Design review of the part built by this model. Coordinates are the model's own, in mm. A direction names the side the tool comes from. Give positions to 0.01 mm unless a question says otherwise; leave off trailing zeros. Order: outer loops, then holes, each group sorted by start corner. A loop starts at its lowest first (then second) coordinate and runs counter-clockwise, first axis right, second up.
```python
from build123d import *

# Parameters (mm, degrees)
BOSS_EXTRUDE1_DEPTH          = 75
SKETCH2_R                    = 2
CUT_EXTRUDE1_DEPTH           = 15
SKETCH4_R                    = 2
CUT_EXTRUDE2_DEPTH           = 12
SKETCH3_R                    = 2.3876
CUT_EXTRUDE3_DEPTH           = 6.35
CUT_EXTRUDE3_DRAFT           = -8
CUT_EXTRUDE3_PROFILE_2_DEPTH = 6.35
CUT_EXTRUDE3_PROFILE_2_DRAFT = -8
CUT_EXTRUDE4_START           = -3
CUT_EXTRUDE4_DEPTH           = 3
CUT_EXTRUDE5_START           = -3
CUT_EXTRUDE5_DEPTH           = 3
CUT_EXTRUDE6_START           = -3
CUT_EXTRUDE6_DEPTH           = 3
CUT_EXTRUDE7_START           = -3
CUT_EXTRUDE7_DEPTH           = 3
SKETCH9_R                    = 1.4951657
CUT_EXTRUDE8_DEPTH           = 5
MIRROR2_COPY_1_SKETCH_R      = 2.3876
MIRROR2_COPY_1_DEPTH         = 6.35
MIRROR2_COPY_1_DRAFT         = -8
MIRROR2_COPY_2_SKETCH_R      = 2.3876
MIRROR2_COPY_2_DEPTH         = 6.35
MIRROR2_COPY_2_DRAFT         = -8
MIRROR2_COPY_3_SKETCH_R      = 2.3876
MIRROR2_COPY_3_DEPTH         = 6.35
MIRROR2_COPY_3_DRAFT         = -8
FILLET2_START                = 5.175
FILLET2_DEPTH                = 42.1845
FILLET2_START_2              = 10.175
FILLET2_2_DEPTH              = 3.491666667
FILLET2_3_DEPTH              = 37.825
FILLET3_R                    = 2


with BuildPart() as part:
    # Sketch1 → Boss-Extrude1 (new body)
    with BuildSketch(Plane(origin=(0, 0, 0), x_dir=(1, 0, 0), z_dir=(0, 1, 0))):
        with BuildLine():
            Line((-6.825, -6.666666667), (-6.825, -25.333333333))
            Line((-6.825, -25.333333333), (8.175, -25.333333333))
            Line((8.175, -25.333333333), (8.175, -13.175))
            Line((8.175, -13.175), (55, -13.175))
            Line((55, -13.175), (55, -1.175))
            Line((55, -1.175), (25, -1.175))
            Line((25, -1.175), (25, 2))
            ThreePointArc((25, 2), (14.923352523, 3.572976633), (5.805515239, 8.142235123))
            ThreePointArc((5.805515239, 8.142235123), (3.047757271, 9.524241472), (0, 10))
            ThreePointArc((0, 10), (-7.071067812, 7.071067812), (-10, 0))
            Line((-10, 0), (-10, -6.666666667))
            Line((-10, -6.666666667), (-6.825, -6.666666667))
        make_face()
    extrude(amount=BOSS_EXTRUDE1_DEPTH)

    # Sketch2 → Cut-Extrude1 (cut)
    with BuildSketch(Plane.ZY.offset(6.825)):
        with Locations((15.666666667, 65)):
            Circle(SKETCH2_R)
    cut_extrude1 = extrude(amount=-CUT_EXTRUDE1_DEPTH, mode=Mode.SUBTRACT)

    # Sketch4 → Cut-Extrude2 (cut)
    with BuildSketch(Plane(origin=(0, 0, 1.175), x_dir=(-1, 0, 0), z_dir=(0, 0, -1))):
        with Locations((-45, 65)):
            Circle(SKETCH4_R)
    cut_extrude2 = extrude(amount=-CUT_EXTRUDE2_DEPTH, mode=Mode.SUBTRACT)


with BuildPart() as cut_extrude3_tool:
    # Sketch3 → Cut-Extrude3 (with draft: the straight prism first)
    with BuildSketch(Plane(origin=(0, 75, 0), x_dir=(1, 0, 0), z_dir=(0, 1, 0))):
        with Locations((1, -1)):
            Circle(SKETCH3_R)
    extrude(amount=-CUT_EXTRUDE3_DEPTH)
    # Cut-Extrude3: the draft: its side faces are tilted about the plane it starts from
    cut_extrude3_sides = [cut_extrude3_tool.faces().sort_by_distance(p)[0] for p in [
        (-1.3876, 71.825, 1),
    ]]
    draft(cut_extrude3_sides, Plane(origin=(0, 75, 0), x_dir=(1, 0, 0), z_dir=(0, 1, 0)), CUT_EXTRUDE3_DRAFT)


with BuildPart() as part_1:
    add(part.part)

    # Cut-Extrude3: cut by cut_extrude3_tool
    add(cut_extrude3_tool.part, mode=Mode.SUBTRACT)


with BuildPart() as cut_extrude3_profile_2_tool:
    # Sketch3 → Cut-Extrude3 profile 2 (with draft: the straight prism first)
    with BuildSketch(Plane(origin=(0, 75, 0), x_dir=(1, 0, 0), z_dir=(0, 1, 0))):
        with Locations((30, -7.175)):
            Circle(SKETCH3_R)
    extrude(amount=-CUT_EXTRUDE3_PROFILE_2_DEPTH)
    # Cut-Extrude3 profile 2: the draft: its side faces are tilted about the plane it starts from
    cut_extrude3_profile_2_sides = [cut_extrude3_profile_2_tool.faces().sort_by_distance(p)[0] for p in [
        (27.6124, 71.825, 7.175),
    ]]
    draft(cut_extrude3_profile_2_sides, Plane(origin=(0, 75, 0), x_dir=(1, 0, 0), z_dir=(0, 1, 0)), CUT_EXTRUDE3_PROFILE_2_DRAFT)


with BuildPart() as part_2:
    add(part_1.part)

    # Cut-Extrude3 profile 2: cut by cut_extrude3_profile_2_tool
    add(cut_extrude3_profile_2_tool.part, mode=Mode.SUBTRACT)

    # Sketch5 → Cut-Extrude4 (cut)
    with BuildSketch(Plane(origin=(8.175, 0, 0), x_dir=(0, 0, -1), z_dir=(1, 0, 0)).offset(CUT_EXTRUDE4_START)):
        Polygon((-19.885416667, 62.564303552), (-15.666666667, 60.128607104), (-11.447916667, 62.564303552), (-11.447916667, 75), (-19.885416667, 75), align=None)
    cut_extrude4 = extrude(amount=-CUT_EXTRUDE4_DEPTH, mode=Mode.SUBTRACT)

    # Sketch6 → Cut-Extrude5 (cut)
    with BuildSketch(Plane(origin=(8.175, 0, 0), x_dir=(0, 0, -1), z_dir=(1, 0, 0)).offset(CUT_EXTRUDE5_START)):
        with BuildLine():
            Line((-13.666666667, 65), (-13.666666667, 75))
            Line((-13.666666667, 75), (-17.666666667, 75))
            Line((-17.666666667, 75), (-17.666666667, 65))
            ThreePointArc((-17.666666667, 65), (-15.666666667, 67), (-13.666666667, 65))
        make_face()
    cut_extrude5 = extrude(amount=CUT_EXTRUDE5_DEPTH, mode=Mode.SUBTRACT)

    # Sketch7 → Cut-Extrude6 (cut)
    with BuildSketch(Plane.XY.offset(13.175).offset(CUT_EXTRUDE6_START)):
        Polygon((40.78125, 62.564303552), (45, 60.128607104), (49.21875, 62.564303552), (49.21875, 75), (40.78125, 75), align=None)
    cut_extrude6 = extrude(amount=-CUT_EXTRUDE6_DEPTH, mode=Mode.SUBTRACT)

    # Sketch8 → Cut-Extrude7 (cut)
    with BuildSketch(Plane.XY.offset(13.175).offset(CUT_EXTRUDE7_START)):
        with BuildLine():
            Line((47, 65), (47, 75))
            Line((47, 75), (43, 75))
            Line((43, 75), (43, 65))
            ThreePointArc((43, 65), (45, 67), (47, 65))
        make_face()
    cut_extrude7 = extrude(amount=CUT_EXTRUDE7_DEPTH, mode=Mode.SUBTRACT)

    # Sketch9 → Cut-Extrude8 (cut)
    with BuildSketch(Plane(origin=(0, 68.65, 0), x_dir=(1, 0, 0), z_dir=(0, 1, 0))):
        with Locations(Location((1, -1, 0), (0, 0, 270))):
            Circle(SKETCH9_R)
        with Locations(Location((30, -7.175, 0), (0, 0, 270))):
            Circle(SKETCH9_R)
    cut_extrude8 = extrude(amount=-CUT_EXTRUDE8_DEPTH, mode=Mode.SUBTRACT)

    # Mirror2: Cut-Extrude1, Cut-Extrude2, Cut-Extrude4, Cut-Extrude5, Cut-Extrude6, Cut-Extrude7, Cut-Extrude8 across plane
    add(cut_extrude1.mirror(Plane.ZX.offset(37.5)), mode=Mode.SUBTRACT)
    add(cut_extrude2.mirror(Plane.ZX.offset(37.5)), mode=Mode.SUBTRACT)
    add(cut_extrude4.mirror(Plane.ZX.offset(37.5)), mode=Mode.SUBTRACT)
    add(cut_extrude5.mirror(Plane.ZX.offset(37.5)), mode=Mode.SUBTRACT)
    add(cut_extrude6.mirror(Plane.ZX.offset(37.5)), mode=Mode.SUBTRACT)
    add(cut_extrude7.mirror(Plane.ZX.offset(37.5)), mode=Mode.SUBTRACT)
    add(cut_extrude8.mirror(Plane.ZX.offset(37.5)), mode=Mode.SUBTRACT)


with BuildPart() as mirror2_copy_1_tool:
    # Mirror2 copy 1 sketch → Mirror2 copy 1 (with draft: the straight prism first)
    with BuildSketch(Plane.XZ):
        with Locations((1, 1)):
            Circle(MIRROR2_COPY_1_SKETCH_R)
    extrude(amount=-MIRROR2_COPY_1_DEPTH)
    # Mirror2 copy 1: the draft: its side faces are tilted about the plane it starts from
    mirror2_copy_1_sides = [mirror2_copy_1_tool.faces().sort_by_distance(p)[0] for p in [
        (-1.3876, 3.175, 1),
    ]]
    draft(mirror2_copy_1_sides, Plane.XZ, MIRROR2_COPY_1_DRAFT)


with BuildPart() as part_3:
    add(part_2.part)

    # Mirror2 copy 1: cut by mirror2_copy_1_tool
    add(mirror2_copy_1_tool.part, mode=Mode.SUBTRACT)


with BuildPart() as mirror2_copy_2_tool:
    # Mirror2 copy 2 sketch → Mirror2 copy 2 (with draft: the straight prism first)
    with BuildSketch(Plane.XZ):
        with Locations((30, 7.175)):
            Circle(MIRROR2_COPY_2_SKETCH_R)
    extrude(amount=-MIRROR2_COPY_2_DEPTH)
    # Mirror2 copy 2: the draft: its side faces are tilted about the plane it starts from
    mirror2_copy_2_sides = [mirror2_copy_2_tool.faces().sort_by_distance(p)[0] for p in [
        (27.6124, 3.175, 7.175),
    ]]
    draft(mirror2_copy_2_sides, Plane.XZ, MIRROR2_COPY_2_DRAFT)


with BuildPart() as part_4:
    add(part_3.part)

    # Mirror2 copy 2: cut by mirror2_copy_2_tool
    add(mirror2_copy_2_tool.part, mode=Mode.SUBTRACT)


with BuildPart() as mirror2_copy_3_tool:
    # Mirror2 copy 3 sketch → Mirror2 copy 3 (with draft: the straight prism first)
    with BuildSketch(Plane.XZ):
        with Locations((30, 7.175)):
            Circle(MIRROR2_COPY_3_SKETCH_R)
    extrude(amount=-MIRROR2_COPY_3_DEPTH)
    # Mirror2 copy 3: the draft: its side faces are tilted about the plane it starts from
    mirror2_copy_3_sides = [mirror2_copy_3_tool.faces().sort_by_distance(p)[0] for p in [
        (27.6124, 3.175, 7.175),
    ]]
    draft(mirror2_copy_3_sides, Plane.XZ, MIRROR2_COPY_3_DRAFT)


with BuildPart() as part_5:
    add(part_4.part)

    # Mirror2 copy 3: cut by mirror2_copy_3_tool
    add(mirror2_copy_3_tool.part, mode=Mode.SUBTRACT)

    # Fillet2: read off the stored shape, not the designer's step
    # Fillet2 outline → Fillet2 (cut)
    with BuildSketch(Plane.YZ.offset(FILLET2_START)):
        with BuildLine():
            Line((1, 13.666666667), (0, 13.666666667))
            Line((0, 13.666666667), (0, 12.666666667))
            ThreePointArc((0, 12.666666667), (0.292893219, 13.373773448), (1, 13.666666667))
        make_face()
        with BuildLine():
            ThreePointArc((1, 17.666666667), (0.292893218, 17.959559886), (0, 18.666666667))
            Line((0, 18.666666667), (0, 17.666666667))
            Line((0, 17.666666667), (1, 17.666666667))
        make_face()
    extrude(amount=FILLET2_DEPTH, mode=Mode.SUBTRACT)

    # Fillet2 2 outline → Fillet2 2 (cut)
    with BuildSketch(Plane.XY.offset(FILLET2_START_2)):
        with BuildLine():
            Line((47, 1), (47, 0))
            Line((47, 0), (47.3595, 0))
            Line((47.3595, 0), (48, 0))
            ThreePointArc((48, 0), (47.292893219, 0.292893219), (47, 1))
        make_face()
        with BuildLine():
            Line((48, 75), (47, 75))
            Line((47, 75), (47, 74))
            ThreePointArc((47, 74), (47.292893219, 74.707106781), (48, 75))
        make_face()
        with BuildLine():
            Line((43, 75), (42, 75))
            ThreePointArc((42, 75), (42.707106781, 74.707106781), (43, 74))
            Line((43, 74), (43, 75))
        make_face()
        with BuildLine():
            ThreePointArc((43, 1), (42.707106781, 0.292893219), (42, 0))
            Line((42, 0), (43, 0))
            Line((43, 0), (43, 1))
        make_face()
    extrude(amount=FILLET2_2_DEPTH, mode=Mode.SUBTRACT)

    # Fillet2 3 outline → Fillet2 3 (cut)
    with BuildSketch(Plane.YZ.offset(FILLET2_START)):
        with BuildLine():
            Line((74, 17.666666667), (75, 17.666666667))
            Line((75, 17.666666667), (75, 18.666666667))
            ThreePointArc((75, 18.666666667), (74.707106782, 17.959559886), (74, 17.666666667))
        make_face()
        with BuildLine():
            Line((75, 12.666666667), (75, 13.666666667))
            Line((75, 13.666666667), (74, 13.666666667))
            ThreePointArc((74, 13.666666667), (74.707106781, 13.373773448), (75, 12.666666667))
        make_face()
    extrude(amount=FILLET2_3_DEPTH, mode=Mode.SUBTRACT)

    # Fillet3
    fillet3_edges = [part_5.edges().sort_by_distance(p)[0] for p in [
        (55, 0, 7.175),
        (0.675, 0, 25.333333333),
        (55, 37.5, 1.175),
        (55, 37.5, 13.175),
        (8.175, 37.5, 25.333333333),
        (-6.825, 37.5, 25.333333333),
        (0.675, 75, 25.333333333),
        (55, 75, 7.175),
    ]]
    fillet(fillet3_edges, radius=FILLET3_R)


solid = part_5.part
```
1. For pin 1 (5 mm diameter, centred on y = 10, z = 15.67, fed in from -X) (3 decimals); pin 2 (9.5 mm diameter, centred on x = 47, y = 6, fed in from +Z) (3 decimals); pin 3 (3 mm diameter, centred on x = 14, y = 48, fed in from -Z), all flat-tipped, find the tip position at first contact; note any pin that passes through.
Recorded:
pin 1: stops at x = -6.825
pin 2: stops at z = 13.175
pin 3: stops at z = -4.45
2. Take a section at D-D (x = 36.5). State the section outline as (y, z) points (3 decimals), then the cut area to 3 significant figures.
Recorded:
outline: (0, 1.175) - (75, 1.175) - (75, 12.667) arc R1 ccw to (74.861, 13.175) - (0.139, 13.175) arc R1 ccw to (0, 12.667) - close
area: 900 mm2
3. Draft analysis for pull direction X (two halves, no side actions). For faces 1 (the face through (31.858, 3.131, 7.76)), 2 (the face through (25, 37, 0)), 3 (the face through (1, 37, 25.333)), state which applies: pulls with the +X half, pulls with the -X half, needs draft (parallel to the pull), parting line crosses it, or undercut.
Recorded:
face 1: undercut
face 2: pulls with the +X half
face 3: needs draft
4. Take a section at C-C (x = 1). State the section outline as (y, z) points, then the cut area to 3 significant figures.
Recorded:
outline: (0, -9.95) - (75, -9.95) - (75, -1.39) - (68.65, -0.5) - (63.65, -0.5) - (63.65, 2.5) - (68.65, 2.5) - (75, 3.39) - (75, 23.33) arc R2 ccw to (73, 25.33) - (2, 25.33) arc R2 ccw to (0, 23.33) - (0, 3.39) - (6.35, 2.5) - (11.35, 2.5) - (11.35, -0.5) - (6.35, -0.5) - (0, -1.39) - close; hole circle Ø4 at (10, 15.67); hole circle Ø4 at (65, 15.67)
area: 2,540 mm2
5. Take a section at A-A (y = 27). State the section outline as (x, z) points (1 decimal).
Recorded:
outline: (-10, 0) arc R10 ccw to (5.8, -8.1) arc R33.1 cw to (25, -2) - (25, 1.2) - (53, 1.2) arc R2 ccw to (55, 3.2) - (55, 11.2) arc R2 ccw to (53, 13.2) - (8.2, 13.2) - (8.2, 23.3) arc R2 ccw to (6.2, 25.3) - (-4.8, 25.3) arc R2 ccw to (-6.8, 23.3) - (-6.8, 6.7) - (-10, 6.7) - close
6. Machinability: for faces 4 (the face through (43, 5, 12)), 5 (the face through (7, 6, 13.667)), 6 (the face through (8.175, 37, 18)), 7 (the face through (42.861, 61.364, 8.696)), 8 (the face through (5.175, 7, 19)), which of the approach directions +Z, -Z, +X, -X, +Y, -Y give a long, thin tool a straight path to every point of the face, cutting with its end or side? Answer none if there is none.
Recorded:
face 4: +Z, -Y
face 5: +X, -Y
face 6: +Z, +X, +Y, -Y
face 7: +Y
face 8: -Y
7. For line 1 along Y through (x, z) = (-6, 15.5); line 2 along Z through (x, y) = (36.5, 56.5) (3 decimals); line 3 along X through (y, z) = (27, 0.5), list the stretches that pass through material, from the lowest coordinate up.
Recorded:
line 1: y = 0 to 8.01, 11.99 to 63.01, 66.99 to 75
line 2: z = 1.175 to 13.175
line 3: x = -10 to 25
8. Take a section at B-B (x = 44). State the section outline as (y, z) points (3 decimals).
Recorded:
outline: (0, 1.175) - (8.268, 1.175) - (8.268, 7.175) - (0, 7.175) - close; (11.732, 1.175) - (63.268, 1.175) - (63.268, 7.175) - (60.706, 7.175) - (60.706, 10.175) - (63.268, 10.175) - (63.268, 13.175) - (11.732, 13.175) - (11.732, 10.175) - (14.294, 10.175) - (14.294, 7.175) - (11.732, 7.175) - close; (66.732, 1.175) - (75, 1.175) - (75, 7.175) - (66.732, 7.175) - close
